Autodesk Inventor part; units mm, degrees
ref_plane "YZ Plane" through (0, 0, 0) normal (1, 0, 0) x (0, 1, 0)
ref_plane "XZ Plane" through (0, 0, 0) normal (0, 1, 0) x (-1, 0, 0)
ref_plane "XY Plane" through (0, 0, 0) normal (0, 0, 1) x (1, 0, 0)
sketch "Sketch1" plane through (0, 0, 0) normal (0, 1, 0) x (-1, 0, 0)
  line L0 (-20, 20) -> (20, 20)
  line L1 (20, 20) -> (20, -20)
  line L2 (20, -20) -> (-20, -20)
  line L3 (-20, -20) -> (-20, 20)
  line L4 (-20, 20) -> (20, -20) construction
  line L5 (20, 20) -> (-20, -20) construction
  line L6 (20, 0) -> (10, 0) construction
  circle A0 centre (10, 0) radius 2.1
  line L7 (10, 0) -> (0, 0) construction
  line L8 (0, 0) -> (-10, 0) construction
  line L9 (-10, 0) -> (-10, -10) construction
  line L10 (-10, -10) -> (-10, 10) construction
  circle A1 centre (-10, 10) radius 2.1
  circle A2 centre (-10, -10) radius 2.1
  dimension "d0" = 40
  dimension "d1" = 40
  dimension "d2" = 10
  dimension "d3" = 4.2
  dimension "d4" = 10
  dimension "d5" = 10
  dimension "d6" = 10
  dimension "d7" = 20
  dimension "d8" = 4.2
  dimension "d9" = 4.2
extrude "Extrusion1" add sketch "Sketch1" along normal blind 20
sketch "Sketch2" plane through (0, 20, 0) normal (0, 1, 0) x (1, 0, 0)
  circle A0 centre (-10, 0) radius 2.1
  circle A1 centre (-10, 0) radius 3
  circle A2 centre (10, 10) radius 2.1
  circle A3 centre (10, 10) radius 3
  circle A4 centre (10, -10) radius 2.1
  circle A5 centre (10, -10) radius 3
  point P0 (0, 0)
  dimension "d12" = 6
  dimension "d13" = 6
  dimension "d14" = 6
extrude "Extrusion2" cut sketch "Sketch2" against normal blind 1 contours A0 | A1 | A2 | A3 | A4 | A5
sketch "Sketch3" plane through (0, 0, 0) normal (0, -1, 0) x (1, 0, 0)
  circle A0 centre (-10, 0) radius 2.1
  circle A1 centre (-10, 0) radius 3
  circle A2 centre (10, 10) radius 3
  circle A3 centre (10, 10) radius 3
  circle A4 centre (10, -10) radius 2.1
  circle A5 centre (10, -10) radius 3
  point P0 (0, 0)
  dimension "d17" = 6
  dimension "d18" = 6
  dimension "d19" = 6
extrude "Extrusion3" cut sketch "Sketch3" against normal blind 1 contours A0 | A1 | A2 | A4 | A5
chamfer "Chamfer1" distance 0.25 angle 45 6 edges at (12.1, 1, 10) (-7.9, 1, 0) (12.1, 1, -10) (12.1, 19, -10) (-7.9, 19, 0) (12.1, 19, 10)
sketch "Sketch4" plane through (-20, 0, -20) normal (-1, 0, 0) x (0, 0, 1)
  line L0 (40, 20) -> (0, 20) construction
  line L1 (20, 20) -> (20, 0) construction
  line L2 (20, 10) -> (27.5, 10) construction
  line L3 (27.5, 10) -> (12.5, 10) construction
  circle A0 centre (12.5, 10) radius 2.1
  circle A1 centre (27.5, 10) radius 2.1
  dimension "d25" = 7.5
  dimension "d26" = 15
  dimension "d27" = 4.2
  dimension "d28" = 4.2
extrude "Extrusion4" cut sketch "Sketch4" against normal blind 15
sketch "Sketch5" plane through (-20, 0, -20) normal (-1, 0, 0) x (0, 0, 1)
  circle A0 centre (12.5, 10) radius 2.1
  circle A1 centre (12.5, 10) radius 3
  circle A2 centre (27.5, 10) radius 2.1
  circle A3 centre (27.5, 10) radius 3
  point P0 (20, 0)
  dimension "d31" = 6
  dimension "d32" = 6
extrude "Extrusion5" cut sketch "Sketch5" against normal blind 1 contours A0 | A1 | A2 | A3
chamfer "Chamfer2" distance 0.25 angle 45 2 edges at (-19, 10, -9.6) (-19, 10, 5.4)
fillet "Fillet1" radius 2.5 4 edges at (-20, 10, -20) (-20, 10, 20) (20, 10, 20) (20, 10, -20)
sketch "Sketch6" plane through (-20, 0, -17.5) normal (-1, 0, 0) x (0, 0, 1)
  line L0 (14.5, 20) -> (20.5, 20) construction
  line L1 (17.5, 20) -> (17.5, 0) construction
  circle A0 centre (17.5, 10) radius 2.1
  line L2 (17.5, 10) -> (32.5, 10) construction
  line L3 (35, 20) -> (35, 0)
  circle A1 centre (32.5, 10) radius 2.1
  line L4 (17.5, 10) -> (2.5, 10) construction
  circle A2 centre (2.5, 10) radius 2.1
  dimension "d39" = 4.2
  dimension "d40" = 15
  dimension "d41" = 4.2
  dimension "d43" = 15
  dimension "d44" = 4.2
extrude "Extrusion6" cut sketch "Sketch6" against normal up to surface (15 mm away)
sketch "Sketch7" plane through (-20, 0, -17.5) normal (-1, 0, 0) x (0, 0, 1)
  circle A0 centre (2.5, 10) radius 2.1
  circle A1 centre (2.5, 10) radius 3
  circle A2 centre (17.5, 10) radius 2.1
  circle A3 centre (17.5, 10) radius 3
  circle A4 centre (32.5, 10) radius 2.1
  circle A5 centre (32.5, 10) radius 3
  point P0 (17.5, 0)
  dimension "d47" = 6
  dimension "d48" = 6
  dimension "d49" = 6
extrude "Extrusion7" cut sketch "Sketch7" against normal blind 1 contours A0 | A1 | A3 | A4 | A5
properties part number "Tool_Holder" material "ABS Plastic"
Here's how the part is built. I have some questions about the finished solid (model axes, mm). A direction names the side the tool comes from. Coordinates: 2 decimals unless noted, no trailing zeros. Write each loop counter-clockwise with the first axis right and the second up, starting at its lowest first coordinate (ties: lowest second). Pieces come first, ordered by that corner, then holes. Notation, with made-up numbers: M -28,84 L -14,84 A27 cw -14,123 Z; hole C 9.25,16.25 d10. An arc over 180 degrees is marked long. Answer as CSV lines item,"result". Start each with the question number.
Q1. Suppose I cut it at D-D, the plane x = 10. State how many separate pieces and enclosed holes the cut face has, then the cut area to 3 significant figures.
Q2. Suppose I cut it at B-B, the plane y = 6. List the corners of the cut face in (x, z) for me.
Q3. For faces 1 (the cylindrical face through (-19.5, 8.2, 12.6)), 2 (the flat face through (-12, 19, 2)), 3 (the flat face through (8, 1, 8)), which set-ups out of +Z, -Z, +X, -X, +Y, -Y let a thin tool reach every point of the face, with its end or its side?
Q4. If we mould it in two halves opening along X, with no side actions, what happens to faces 4 (the flat face through (-19, 8, 16.3)), 5 (the flat face through (8, 1, -12)), 6 (the flat face through (0, 0, 0)), 7 (the cylindrical face through (-12.4, 0.5, -1.8))? For each: pulls with the +X half, pulls with the -X half, needs draft (parallel to the pull), parting line crosses it, or undercut.
Q5. I need wall thicknesses on probe 1 along Z at (x, y) = (10, 8.75); probe 2 along Z at (x, y) = (-10, 19.6); probe 3 along X at (y, z) = (19.85, 0). Which ranges of each line are inside material? Lowest first, please. Write a range as [from, to].
Q6. Suppose I cut it at A-A, the plane x = -16. List the corners of the cut face in (y, z) for me.
Q7. Suppose I cut it at C-C, the plane z = -15. List the corners of the cut face in (x, y) for me, then the cut area to 3 significant figures.
Q8. Will these pins go through, and if not, where does the flat tip stop? pin 1 Ø5 at (x, z) = (10, -10) entering from -Y; pin 2 Ø5 at (y, z) = (10, 0) entering from -X; pin 3 Ø5 at (x, z) = (10, -10) entering from +Y.
Entries:
1,separate pieces,"3"
1,enclosed holes,"0"
1,area,"625 mm²"
2,outline,"M -20,-17.5 A2.5 ccw -17.5,-20 L 17.5,-20 A2.5 ccw 20,-17.5 L 20,17.5 A2.5 ccw 17.5,20 L -17.5,20 A2.5 ccw -20,17.5 Z; hole C -10,0 d4.2; hole C 10,-10 d4.2; hole C 10,10 d4.2"
3,face 1,"-X"
3,face 2,"+Y"
3,face 3,"-Y"
4,face 4,"pulls with the -X half"
4,face 5,"undercut"
4,face 6,"needs draft"
4,face 7,"undercut"
5,probe 1,"z = [-20, -12.1], [-7.9, 7.9], [12.1, 20]"
5,probe 2,"z = [-20, -3], [3, 20]"
5,probe 3,"x = [-20, -13], [-7, 20]"
6,outline,"M 0,-20 L 20,-20 L 20,20 L 0,20 Z; hole C 10,-15 d4.2; hole C 10,-7.5 d4.2; hole C 10,0 d4.2; hole C 10,7.5 d4.2; hole C 10,15 d4.2"
7,outline,"M -20,0 L 20,0 L 20,20 L -20,20 L -20,13 L -19,13 L -19,12.1 L -5,12.1 L -5,7.9 L -19,7.9 L -19,7 L -20,7 Z"
7,area,"735 mm²"
8,pin 1,"stops at y = 1"
8,pin 2,"stops at x = -19"
8,pin 3,"stops at y = 19"
